Source: CAD feature listing. Evaluate the final solid. Frame: model axes, mm. A direction names the side the tool comes from. Give positions to 0.01 mm unless a question says otherwise; leave off trailing zeros. Loops run counter-clockwise (first coordinate to the right, second up) from the corner with the lowest first, then second, coordinate; pieces in that order, holes last. Notation, with made-up numbers: (-17, -31.5) -> (-2, -31.5) arc R15 ccw to (-2, -19.5) -> close; hole circle Ø3 at (61, 27.25). An arc over 180 degrees is marked (long way). Return JSON: item names as keys, results as strings. Group by question number.
Autodesk Inventor part; units mm, degrees
ref_plane "YZ Plane" through (0, 0, 0) normal (1, 0, 0) x (0, 1, 0)
ref_plane "XZ Plane" through (0, 0, 0) normal (0, 1, 0) x (-1, 0, 0)
ref_plane "XY Plane" through (0, 0, 0) normal (0, 0, 1) x (1, 0, 0)
sketch "草图1" plane through (0, 0, 0) normal (0, 0, 1) x (1, 0, 0)
  line L0 (0, 0) -> (0, 30)
  line L1 (0, 30) -> (-16, 30)
  line L2 (-16, 30) -> (-16, 26)
  line L3 (-16, 26) -> (-55, 26)
  line L4 (-54.8586, 22.861) -> (-50.0487, 20.9752)
  line L5 (-50.0487, 20.9752) -> (-50.0487, 17.9752)
  line L6 (-50.0487, 17.9752) -> (-55, 16.5)
  line L7 (0, 0) -> (-16, 0)
  line L8 (-16, 0) -> (-16, 4)
  line L9 (-16, 4) -> (-55, 4)
  line L10 (-55, 13.5) -> (-50.0487, 12.0248)
  line L11 (-50.0487, 12.0248) -> (-50.0487, 9.0248)
  line L12 (-50.0487, 9.0248) -> (-54.8586, 7.139)
  line L13 (-55, 16.5) -> (-55, 13.5)
  line L14 (-54.8586, 4) -> (-54.8586, 7.139)
  line L15 (-54.8586, 26) -> (-54.8586, 22.861)
  point P0 (-54.9901, 12.2219)
  dimension "d0" = 30
  dimension "d1" = 16
  dimension "d2" = 4
  dimension "d3" = 39
  dimension "d4" = 22
  dimension "d5" = 38
  dimension "d7" = 3
  dimension "d8" = 38
  dimension "d9" = 3
revolve "旋转1" add sketch "草图1" angle 360 about axis through (0, 0, 0) along (0, 1, 0)
sketch "草图2" plane through (0, 26, 0) normal (0, 1, 0) x (1, 0, 0)
  circle A0 centre (0, 0) radius 54.8586
  circle A1 centre (0, 0) radius 16
  circle A2 centre (0, 0) radius 30
  circle A3 centre (0, -30) radius 12
  circle A4 centre (25.9808, -15) radius 12
  circle A5 centre (25.9808, 15) radius 12
  circle A6 centre (0, 30) radius 12
  circle A7 centre (-25.9808, 15) radius 12
  circle A8 centre (-25.9808, -15) radius 12
  dimension "d14" = 24
  dimension "d17" = 360
sketch "草图3" plane through (0, 0, 0) normal (0, -1, 0) x (1, 0, 0)
  circle A0 centre (0, 0) radius 16
  arc A1 (-7.2284, -2) -> (-7.2284, 2) centre (0, 0) ccw
  line L0 (-9.6, 0) -> (-9.6, 2)
  line L1 (-9.6, 2) -> (-9.6, -2)
  line L2 (-9.6, -2) -> (-7.2284, -2)
  line L3 (-9.6, 2) -> (-7.2284, 2)
  dimension "d19" = 15
  dimension "d20" = 9.6
  dimension "d21" = 2
  dimension "d22" = 4
extrude "拉伸1" cut sketch "草图3" against normal through all contours L2 L1 L0 L3 A1
extrude "拉伸2" cut sketch "草图2" against normal blind 8.74 contours A5 A2 | A2 A5 | A4 A2 | A2 A4 | A6 A2 | A2 A6 | A3 A2 | A2 A3 | A7 A2 | A2 A7 | A8 A2 | A2 A8
sketch "草图4" plane through (0, 4, 0) normal (0, -1, 0) x (1, 0, 0)
  circle A0 centre (0, 0) radius 16
  circle A1 centre (-25.9808, -15) radius 12
  circle A2 centre (-25.9808, 15) radius 12
  circle A3 centre (0, 30) radius 12
  point P0 (0, 30)
  point P1 (25.9808, 15)
  point P2 (25.9808, -15)
  point P3 (0, -30)
  point P4 (-25.9808, -15)
  dimension "d29" = 360
hole "孔1" at (-25.9808, 4, 15) at (0, 4, 30) at (25.9808, 4, 15) at (25.9808, 4, -15) at (0, 4, -30) at (-25.9808, 4, -15) direction (0, 1, 0) diameter 24 depth 8.74
properties part number "1"
1) Cut plane B-B on y = 5.75. Return loops of the section in (x, z).
2) Material intervals for line 1 (Z direction, x = 36, y = 24.75); line 2 (X direction, y = 24, z = 15); line 3 (Z direction, x = 18.5, y = 6.5), sorted ascending.
3) Reachability of faces 1 (the face through (10.917, 12.117, -49.161)), 2 (the face through (26, 12.74, -15)), 3 (the face through (-11.42, 26, -11.42)) from +Z, -Z, +X, -X, +Y, -Y: full face, straight path, thin tool, end or side. Return the list, or none.
4) Mould query, pull axis Y, two halves, no side actions, for faces 4 (the face through (11.892, 5.591, -53.554)), 5 (the face through (-48.033, 17.883, -15.126)), 6 (the face through (26, 12.74, 15)). Classes: released by +Y, released by -Y, zero draft, split by the parting line, or undercut.
5) Contact query for flat-ended pins moving along their axis: P1, Ø5, axis at x = -40, z = -6.5, coming from the +Y side; P2, Ø2, axis at x = -43.5, y = 19, coming from the +Z side; P3, Ø1.5, axis at y = 17, z = 23, coming from the -X side. Output: stop coordinate, or through.
Calculated:
{
 "1": {"outline": "circle Ø109.72 at (0, 0); hole circle Ø24 at (-25.98, -15); hole circle Ø24 at (-25.98, 15); hole circle Ø24 at (0, -30); hole circle Ø24 at (0, 30); hole (-9.6, -2) -> (-7.23, -2) arc R7.5 ccw (long way) to (-7.23, 2) -> (-9.6, 2) -> close; hole circle Ø24 at (25.98, -15); hole circle Ø24 at (25.98, 15)"},
 "2": {"line 1": "-41.39 to -21.6, -8.4 to 8.4, 21.6 to 41.39", "line 2": "-52.77 to -37.98, -13.98 to 13.98, 37.98 to 52.77", "line 3": "-51.65 to -24.38, -5.62 to 5.62, 24.38 to 51.65"},
 "3": {"face 1": "none", "face 2": "-Y", "face 3": "+Y"},
 "4": {"face 4": "zero draft", "face 5": "undercut", "face 6": "released by -Y"},
 "5": {"P1": "y = 26", "P2": "z = 26.43", "P3": "x = -50.21"}
}
